The model under review builds one solid part; all positions refer to its coordinate system, in mm. Face numbers are marked on the shaded views. A direction names the side the tool comes from. Coordinates: 2 decimals unless noted, no trailing zeros. Order: outer loops, then holes, each group sorted by start corner. A loop starts at its lowest first (then second) coordinate and runs counter-clockwise, first axis right, second up.
```python
from build123d import *

# Parameters (mm, degrees)
F1_DEPTH = 914.4
F2_R     = 5.08
F3_W     = 904.24
F3_H     = 203.2
F3_W_2   = 701.04
F3_H_2   = 101.6
F3_W_3   = 449.58
F3_H_3   = 543.56
F3_W_4   = 246.38
F3_H_4   = 340.36
F4_DEPTH = 6.35


with BuildPart() as f1:
    # F0 (on Right) → F1 (new body)
    with BuildSketch(Plane.YZ):
        Polygon((-482.6, 0), (0, 0), (0, 914.4), (-609.6, 914.4), (-609.6, 863.6), (-558.8, 863.6), (-558.8, 101.6), (-482.6, 101.6), align=None)
    extrude(amount=F1_DEPTH)

    # F2
    f2_edges = [f1.edges().sort_by_distance(p)[0] for p in [
        (457.2, -609.6, 914.4),
        (457.2, -609.6, 863.6),
    ]]
    fillet(f2_edges, radius=F2_R)

    # F3 (on face) → F4 (join)
    with BuildSketch(Plane.XZ.offset(558.8)):
        with Locations((457.2, 756.92)):
            Rectangle(F3_W, F3_H)
        with Locations((457.2, 756.92)):
            Rectangle(F3_W_2, F3_H_2, mode=Mode.SUBTRACT)
        with Locations((684.53, 378.46)):
            Rectangle(F3_W_3, F3_H_3)
        with Locations((684.53, 378.46)):
            Rectangle(F3_W_4, F3_H_4, mode=Mode.SUBTRACT)
        with Locations((229.87, 378.46)):
            Rectangle(F3_W_3, F3_H_3)
        with Locations((229.87, 378.46)):
            Rectangle(F3_W_4, F3_H_4, mode=Mode.SUBTRACT)
    extrude(amount=F4_DEPTH)


solid = f1.part
```
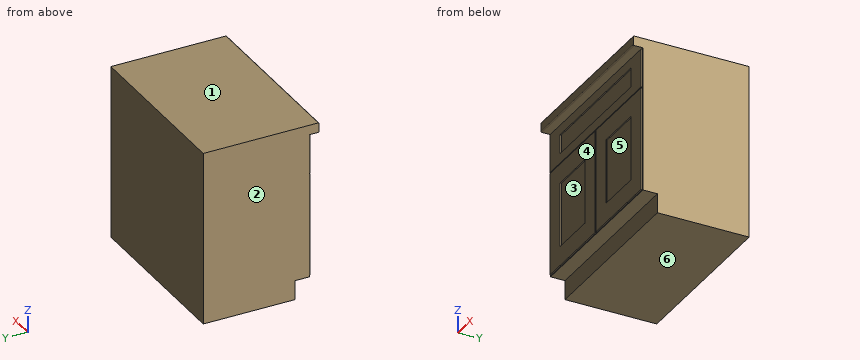
(1) We need section C-C, the plane x = 396. Write out the cut boundary in (y, z).
A:
outline: (-609.6, 868.68) arc R5.08 ccw to (-604.52, 863.6) - (-558.8, 863.6) - (-558.8, 858.52) - (-565.15, 858.52) - (-565.15, 807.72) - (-558.8, 807.72) - (-558.8, 706.12) - (-565.15, 706.12) - (-565.15, 655.32) - (-558.8, 655.32) - (-558.8, 650.24) - (-565.15, 650.24) - (-565.15, 106.68) - (-558.8, 106.68) - (-558.8, 101.6) - (-482.6, 101.6) - (-482.6, 0) - (0, 0) - (0, 914.4) - (-604.52, 914.4) arc R5.08 ccw to (-609.6, 909.32) - close
(2) We need section B-B, the plane x = 707.5. Write out the cut boundary in (y, z), and give its area (3 significant figures).
A:
outline: (-609.6, 868.68) arc R5.08 ccw to (-604.52, 863.6) - (-558.8, 863.6) - (-558.8, 858.52) - (-565.15, 858.52) - (-565.15, 807.72) - (-558.8, 807.72) - (-558.8, 706.12) - (-565.15, 706.12) - (-565.15, 655.32) - (-558.8, 655.32) - (-558.8, 650.24) - (-565.15, 650.24) - (-565.15, 548.64) - (-558.8, 548.64) - (-558.8, 208.28) - (-565.15, 208.28) - (-565.15, 106.68) - (-558.8, 106.68) - (-558.8, 101.6) - (-482.6, 101.6) - (-482.6, 0) - (0, 0) - (0, 914.4) - (-604.52, 914.4) arc R5.08 ccw to (-609.6, 909.32) - close
area: 508,000 mm2
(3) Draft analysis for pull direction X (two halves, no side actions). For the marked faces 1, 2 and 3, state which applies: released by +X, released by -X, zero draft, split by the parting line, or undercut.
A:
face 1: zero draft
face 2: released by -X
face 3: undercut
(4) Wall thickness on probe 1 along Y at (x, z) = (860.5, 50.5); probe 2 along Z at (x, y) = (828, -502); probe 3 along Y at (x, z) = (581.5, 221.5): over which ranges is each line inside the solid? List them lowest first.
A:
probe 1: y = -482.6 to 0
probe 2: z = 101.6 to 914.4
probe 3: y = -558.8 to 0
(5) Machinability: for the marked faces 4, 5 and 6, which of the approach directions +Z, -Z, +X, -X, +Y, -Y give a long, thin tool a straight path to every point of the face, cutting with its end or side? Answer none if there is none.
A:
face 4: -Z, +X, -X, -Y
face 5: -Y
face 6: -Z, +X, -X, +Y, -Y
(6) We need section A-A, the plane z = 324. Write out the cut boundary in (x, y).
A:
outline: (0, -558.8) - (5.08, -558.8) - (5.08, -565.15) - (106.68, -565.15) - (106.68, -558.8) - (353.06, -558.8) - (353.06, -565.15) - (454.66, -565.15) - (454.66, -558.8) - (459.74, -558.8) - (459.74, -565.15) - (561.34, -565.15) - (561.34, -558.8) - (807.72, -558.8) - (807.72, -565.15) - (909.32, -565.15) - (909.32, -558.8) - (914.4, -558.8) - (914.4, 0) - (0, 0) - close
(7) We need section D-D, the plane z = 124.5. Write out the cut boundary in (x, y), and give its area (3 significant figures).
A:
outline: (0, -558.8) - (5.08, -558.8) - (5.08, -565.15) - (454.66, -565.15) - (454.66, -558.8) - (459.74, -558.8) - (459.74, -565.15) - (909.32, -565.15) - (909.32, -558.8) - (914.4, -558.8) - (914.4, 0) - (0, 0) - close
area: 517,000 mm2
(8) For pin 1 Ø3 at (y, z) = (-561.5, 342.5) entering from -X; pin 2 Ø1.9 at (y, z) = (-561, 755.5) entering from +X; pin 3 Ø12 at (x, z) = (292, 218) entering from -Y, all flat-tipped, find the tip position at first contact; note any pin that passes through.
A:
pin 1: stops at x = 5.08
pin 2: stops at x = 909.32
pin 3: stops at y = -558.8
